Part print with two shaded views. Sizes in mm from the minimum x, y, z corner. A direction names the side the tool comes from. Give positions to 0.01 mm unless a question says otherwise; leave off trailing zeros. Write each loop counter-clockwise with the first axis right and the second up, starting at its lowest first coordinate (ties: lowest second). Pieces come first, ordered by that corner, then holes. Notation, with made-up numbers: (-9.5, 36) -> (35.5, 36) arc R13 cw to (35.5, 55) -> close; hole circle Ø3 at (-5.75, 55). An arc over 180 degrees is marked (long way). Answer as a JSON object with one key per item and string values.
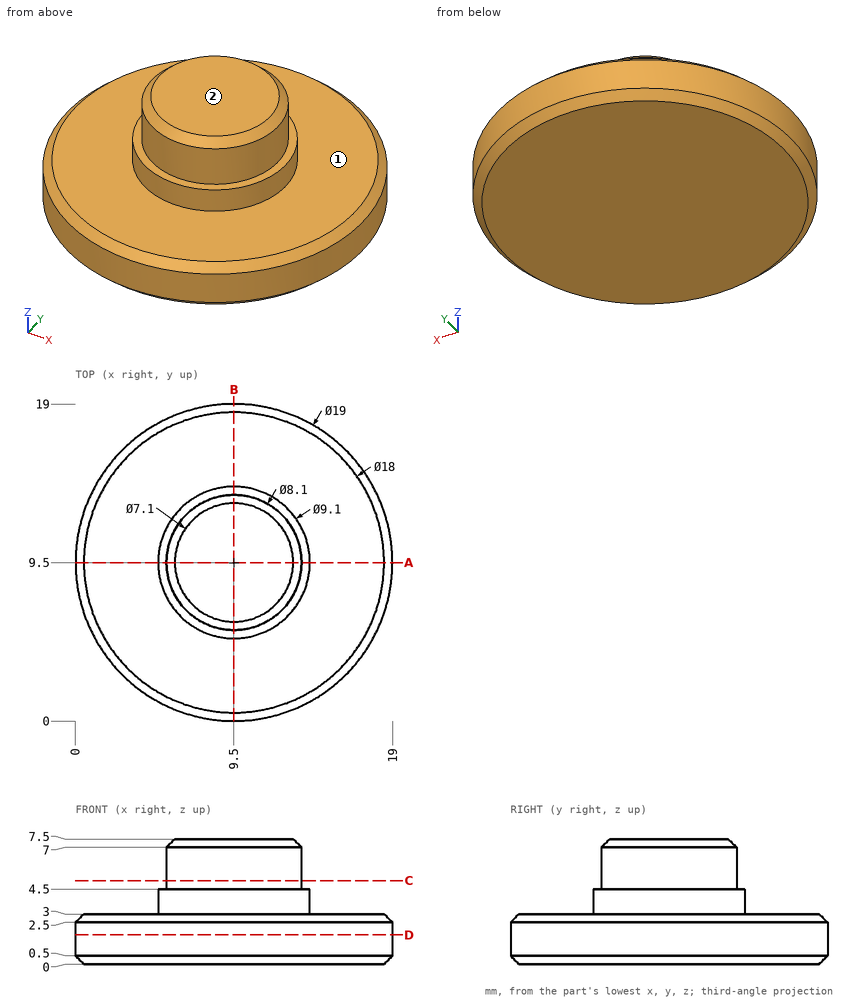
1) Slice it at C-C (z = 5). List the corners of the cut face in (x, y).
Model answer:
{"outline": "circle Ø8.1 at (9.5, 9.5)"}
2) Wall check: probe 1 along Z at (x, y) = (3.75, 4.5); probe 2 along Z at (x, y) = (13.5, 8); probe 3 along Y at (x, z) = (13.5, 2). Give the ranges that are in metal, low to high.
Model answer:
{"probe 1": "z = 0 to 3", "probe 2": "z = 0 to 4.5", "probe 3": "y = 0.88 to 18.12"}
3) 3-axis set-ups, long thin cutter, end or side, ignore diameter. For the marked faces 1 and 2: which of +Z, -Z, +X, -X, +Y, -Y reach the whole face in a straight line?
Model answer:
{"face 1": "+Z", "face 2": "+Z, +X, -X, +Y, -Y"}
4) Pin check, flat tips, straight feed: pin 1 (3 mm diameter, centred on x = 16, z = 2.5, fed in from +Y); pin 2 (4 mm diameter, centred on y = 15, z = 2, fed in from +X); pin 3 (6 mm diameter, centred on x = 17, y = 4.5, fed in from +Z). Stop position of each tip, or through.
Model answer:
{"pin 1": "stops at y = 17.58", "pin 2": "stops at x = 18.33", "pin 3": "stops at z = 3"}
5) Slice it at D-D (z = 1.75). List the corners of the cut face in (x, y), then the cut area to 3 significant figures.
Model answer:
{"outline": "circle Ø19 at (9.5, 9.5)", "area": "284 mm2"}
6) Slice it at A-A (y = 9.5). List the corners of the cut face in (x, z), then the cut area to 3 significant figures.
Model answer:
{"outline": "(0, 0.5) -> (0.5, 0) -> (18.5, 0) -> (19, 0.5) -> (19, 2.5) -> (18.5, 3) -> (14.05, 3) -> (14.05, 4.5) -> (13.55, 4.5) -> (13.55, 7) -> (13.05, 7.5) -> (5.95, 7.5) -> (5.45, 7) -> (5.45, 4.5) -> (4.95, 4.5) -> (4.95, 3) -> (0.5, 3) -> (0, 2.5) -> close", "area": "94.2 mm2"}
